```python
from build123d import *

# Parameters (mm, degrees)
F1_DEPTH = 25


with BuildPart() as f1:
    # F0 (on Front) → F1 (new body)
    with BuildSketch(Plane.XZ):
        Polygon((0, 0), (-48.926342, -74.815616), (51.997956, -74.815616), align=None)
        Polygon((-48.926342, 0), (-48.926342, -74.815616), (0, 0), align=None)
        Polygon((-37.078708, 44.099528), (0, 0), (-15.557691, 65.769808), align=None)
        Polygon((-15.557691, 65.769808), (0, 0), (21.13994, 65.769808), (8.463154, 56.959255), (-9.434227, 56.959255), align=None)
        Polygon((21.13994, 65.769808), (0, 0), (36.201105, 44.099528), align=None)
        Polygon((36.201105, 44.099528), (0, 0), (51.997956, 0), align=None)
        Polygon((0, 0), (51.997956, -74.815616), (51.997956, 0), align=None)
        Polygon((-48.926342, 0), (0, 0), (-37.078708, 44.099528), align=None)
    extrude(amount=F1_DEPTH)


solid = f1.part
```
Could you check a few things on this model? Use its own coordinates, in mm. A direction names the side the tool comes from. Round coordinates to 2 decimals unless told otherwise and drop trailing zeros. Loops run counter-clockwise (first coordinate to the right, second up) from the corner with the lowest first, then second, coordinate; pieces in that order, holes last. Notation, with made-up numbers: M 84,-18.75 L 88,-18.75 A16 ccw 88,3.25 Z; hole C 25,19 d7. An arc over 180 degrees is marked long. Answer as CSV lines item,"result".
1) For pin 1 Ø14.5 at (x, y) = (0.5, -8.5) entering from +Z; pin 2 Ø8 at (y, z) = (-14.5, 19) entering from +X; pin 3 Ø1 at (x, y) = (19.5, -3.5) entering from +Z, each with a flat end and sliding along its axis, tell me the tip position at first contact or that it passes through.
From the geometry:
pin 1,"z = 56.96"
pin 2,"x = 46.62"
pin 3,"z = 64.98"
2) Imagine slicing it at A-A on y = -9. List the corners of the cut face in (x, z) for me, and give its area (3 significant figures).
From the geometry:
outline,"M -48.93,-74.82 L 52,-74.82 L 52,0 L 36.2,44.1 L 21.14,65.77 L 8.46,56.96 L -9.43,56.96 L -15.56,65.77 L -37.08,44.1 L -48.93,0 Z"
area,"12,300 mm^2"
3) If I drill on probe 1 along Z at (x, y) = (5, -4.5); probe 2 along Z at (x, y) = (-34.5, -3.5); probe 3 along X at (y, z) = (-18.5, 19), over which ranges is the centre line in solid material (lowest first)?
From the geometry:
probe 1,"-74.82 to 56.96"
probe 2,"-74.82 to 46.7"
probe 3,"-43.82 to 45.19"
4) Imagine slicing it at C-C on z = 31.5. List the corners of the cut face in (x, y) for me.
From the geometry:
outline,"M -40.46,-25 L 40.71,-25 L 40.71,0 L -40.46,0 Z"
5) Imagine slicing it at B-B on x = 3. List the corners of the cut face in (y, z) for me.
From the geometry:
outline,"M -25,-74.82 L 0,-74.82 L 0,56.96 L -25,56.96 Z"
6) Which directions (+Z, -Z, +X, -X, +Y, -Y) give clear straight access to the entire face, cutting with the end or side of a thin tool? Please do faces 4 (the flat face through (1, -12, -74.816)), 5 (the flat face through (14.89, -12.325, 61.426)).
From the geometry:
face 4,"-Z, +X, -X, +Y, -Y"
face 5,"+Z, +Y, -Y"
7) We'd pull the mould along X, two halves only. Please class faces 1 (the flat face through (-48.926, -12, -37)), 2 (the flat face through (0, -12, 56.959)), 3 (the flat face through (51.998, -12, -38)): released by +X, released by -X, zero draft, split by the parting line, or undercut.
From the geometry:
face 1,"released by -X"
face 2,"undercut"
face 3,"released by +X"
